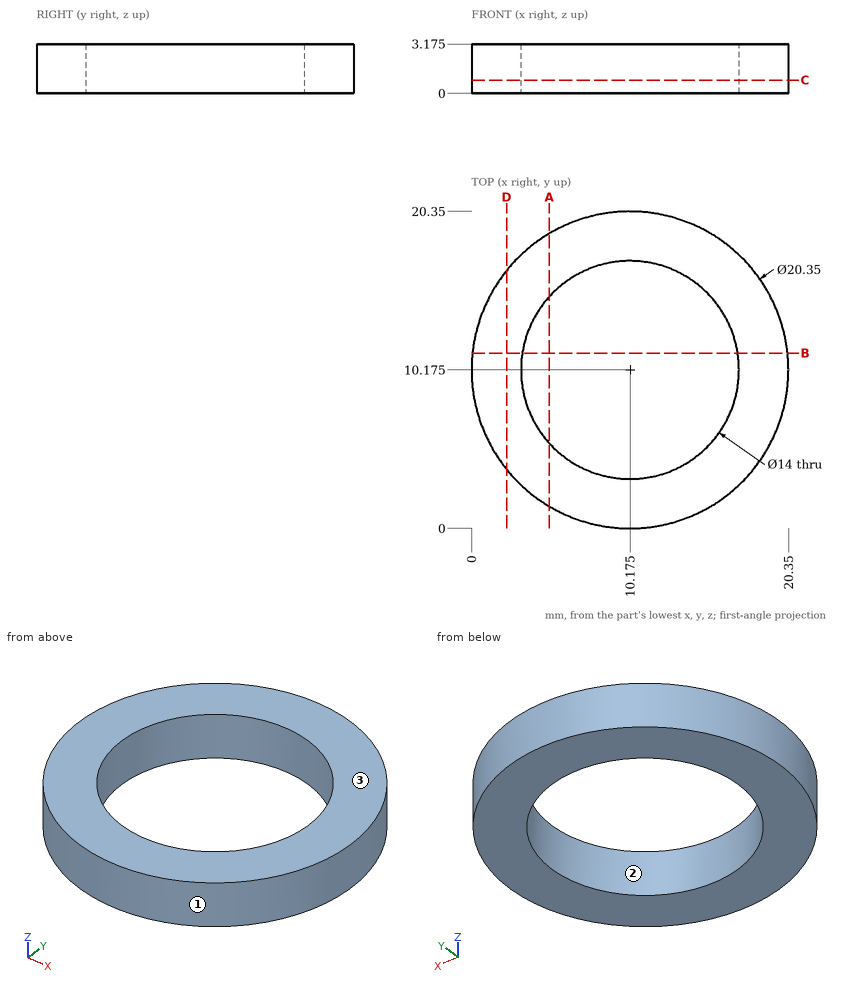
The drawing under review shows one solid part. Ordinate dimensions are in mm from its lowest x, y, z. Coordinates: 2 decimals unless noted, no trailing zeros. Order: outer loops, then holes, each group sorted by start corner. A loop starts at its lowest first (then second) coordinate and runs counter-clockwise, first axis right, second up. Notation, with made-up numbers: (-3, 69) -> (31, 69) arc R9 cw to (31, 76) -> close; hole circle Ø9 at (70, -25.5). An arc over 180 degrees is marked (long way). Use CSV: the item, a comma, the result in double quotes. Start each with the question number.
Item 1: Insertion check: pin 1 (1.5 mm diameter, centred on y = 14, z = 0.5, fed in from -X); pin 2 (8 mm diameter, centred on x = 17, y = 10.5, fed in from +Z) (3 decimals); pin 3 (2 mm diameter, centred on x = 6, y = 6, fed in from -Z); pin 4 (1.5 mm diameter, centred on y = 11.5, z = 1, fed in from +X). Each pin has a flat end and moves straight along its axis. Give the tip position at first contact, or say it passes through.
Item 2: We need section C-C, the plane z = 0.85. Give the boundary of the cut face in (x, y) (3 decimals), then the cut area to 3 significant figures.
Item 3: Draft analysis for pull direction Y (two halves, no side actions). For the marked faces 1, 2 and 3, state which applies: pulls with the +Y half, pulls with the -Y half, needs draft (parallel to the pull), parting line crosses it, or undercut.
Item 4: We need section B-B, the plane y = 11.25. Give the boundary of the cut face in (x, z) (3 decimals), then the cut area to 3 significant figures.
Item 5: We need section D-D, the plane x = 2.25. Give the boundary of the cut face in (y, z) (3 decimals).
Item 6: Wall thickness on probe 1 along Y at (x, z) = (16, 0.6); probe 2 along Y at (x, z) = (5, 2.85): over which ranges is each line inside the solid? List them lowest first.
Item 7: We need section A-A, the plane x = 5. Give the boundary of the cut face in (y, z) (3 decimals).
Derived:
1,pin 1,"stops at x = 0.48"
1,pin 2,"stops at z = 3.175"
1,pin 3,"passes through"
1,pin 4,"stops at x = 20.33"
2,outline,"circle Ø20.35 at (10.175, 10.175); hole circle Ø14 at (10.175, 10.175)"
2,area,"171 mm^2"
3,face 1,"parting line crosses it"
3,face 2,"undercut"
3,face 3,"needs draft"
4,outline,"(0.057, 0) -> (3.258, 0) -> (3.258, 3.175) -> (0.057, 3.175) -> close; (17.092, 0) -> (20.293, 0) -> (20.293, 3.175) -> (17.092, 3.175) -> close"
4,area,"20.3 mm^2"
5,outline,"(3.793, 0) -> (16.557, 0) -> (16.557, 3.175) -> (3.793, 3.175) -> close"
6,probe 1,"y = 1.83 to 6.29, 14.06 to 18.52"
6,probe 2,"y = 1.41 to 5.46, 14.89 to 18.94"
7,outline,"(1.414, 0) -> (5.461, 0) -> (5.461, 3.175) -> (1.414, 3.175) -> close; (14.889, 0) -> (18.936, 0) -> (18.936, 3.175) -> (14.889, 3.175) -> close"
